from build123d import *

# Parameters (mm, degrees)
BASPROSKE_W         = 4
BASPROSKE_H         = 7.875
TOOTHCUT_DEPTH      = 12.833480046
TEETHCUTS_COUNT     = 12
TEETHCUTS_ANGLE     = 330
BORSKE_R            = 1
BORE_DEPTH          = 50.0000508
SKETCH1_R           = 3.25
SKETCH1_R_2         = 2.25
BOSS_EXTRUDE1_DEPTH = 2
SKETCH2_R           = 2
CUT_EXTRUDE1_DEPTH  = 3


with BuildPart() as part:
    # BasProSke → Base-Revolve (revolve)
    with BuildSketch(Plane(origin=(0, 0, 0), x_dir=(1, 0, 0), z_dir=(0, 1, 0)), mode=Mode.PRIVATE) as base_revolve_sk:
        with Locations((2, 3.9375)):
            Rectangle(BASPROSKE_W, BASPROSKE_H)
    revolve(base_revolve_sk.sketch.rotate(Axis((-10, 0, 0), (1, 0, 0)), 180), axis=Axis((-10, 0, 0), (1, 0, 0)))

    # TooCutSke → ToothCut (cut, through all)
    with BuildSketch(Plane(origin=(0, 0, 0), x_dir=(0, 0, -1), z_dir=(1, 0, 0))):
        with BuildLine():
            ThreePointArc((0.631439839, 5.305305014), (0, 5.34275), (-0.631439839, 5.305305014))
            ThreePointArc((-0.631439839, 5.305305014), (-0.93992237, 6.654932089), (-1.876748184, 7.674251521))
            ThreePointArc((-1.876748184, 7.674251521), (0, 7.9004), (1.876748184, 7.674251521))
            ThreePointArc((1.876748184, 7.674251521), (0.93992237, 6.654932089), (0.631439839, 5.305305014))
        make_face()
    toothcut = extrude(amount=TOOTHCUT_DEPTH, mode=Mode.SUBTRACT)

    # TeethCuts: ToothCut ×12 about axis
    teethcuts_axis = Axis((-10, 0, 0), (1, 0, 0))
    for i in range(1, TEETHCUTS_COUNT):
        add(toothcut.rotate(teethcuts_axis, i * TEETHCUTS_ANGLE / (TEETHCUTS_COUNT - 1)), mode=Mode.SUBTRACT)

    # BorSke → Bore (cut, symmetric)
    with BuildSketch(Plane(origin=(0, 0, 0), x_dir=(0, 0, -1), z_dir=(1, 0, 0))):
        with Locations(Location((0, 0, 0), (0, 0, 180))):
            Circle(BORSKE_R)
    extrude(amount=BORE_DEPTH, both=True, mode=Mode.SUBTRACT)

    # Sketch1 → Boss-Extrude1 (add)
    with BuildSketch(Plane.ZY):
        with Locations(Location((0, 0, 0), (0, 0, 180))):
            Circle(SKETCH1_R)
        Circle(SKETCH1_R_2, mode=Mode.SUBTRACT)
    extrude(amount=BOSS_EXTRUDE1_DEPTH)

    # Sketch2 → Cut-Extrude1 (cut)
    with BuildSketch(Plane(origin=(4, 0, 0), x_dir=(0, 0, -1), z_dir=(1, 0, 0))):
        Circle(SKETCH2_R)
    extrude(amount=-CUT_EXTRUDE1_DEPTH, mode=Mode.SUBTRACT)


solid = part.part
Could you check a few things on this model? Use its own coordinates, in mm. A direction names the side the tool comes from. Give positions to 0.01 mm unless a question says otherwise; leave off trailing zeros. Order: outer loops, then holes, each group sorted by start corner. A loop starts at its lowest first (then second) coordinate and runs counter-clockwise, first axis right, second up. Notation, with made-up numbers: (17, -19) -> (55, -19) arc R18 cw to (55, 10) -> close; hole circle Ø2 at (16.5, -1). An arc over 180 degrees is marked (long way). Answer in a Markdown table with one row per item. Add a question column.
Item 1: Imagine slicing it at A-A (z = 0). List the corners of the cut face in (x, y) for me.
Item 2: I'm going to push flat-ended pins straight in: P1, Ø8, axis at y = 0, z = -5, coming from the -X side; P2, Ø2, axis at y = 0.5, z = -0.5, coming from the +X side. Where does each tip first touch, or does it pass through?
Item 3: Please list where these lines run through material, in increasing order: probe 1 along Y at (x, z) = (-0.8, 0); probe 2 along Z at (x, y) = (3.2, -5); probe 3 along Y at (x, z) = (2.55, 0).
Item 4: Imagine slicing it at D-D (z = 6.75). List the corners of the cut face in (x, y) for me.
Item 5: Imagine slicing it at C-C (x = -0.8). List the corners of the cut face in (y, z) for me.
Item 6: We'd pull the mould along Y, two halves only. Please class faces 1 (the cylindrical face through (1.97, -2.51, -6.2)), 2 (the cylindrical face through (-0.986, 1.978, 2.579)): pulls with the +Y half, pulls with the -Y half, needs draft (parallel to the pull), parting line crosses it, or undercut.
Item 7: For faces 3 (the cylindrical face through (1.972, -6.235, -2.514)), 4 (the flat face through (1, -1, -1)), which set-ups out of +Z, -Z, +X, -X, +Y, -Y let a thin tool reach every point of the face, with its end or its side?
Result:
| question | item | result |
|---|---|---|
| 1 | outline | (-2, -3.25) -> (0, -3.25) -> (0, -5.34) -> (4, -5.34) -> (4, -2) -> (1, -2) -> (1, -1) -> (0, -1) -> (0, -2.25) -> (-2, -2.25) -> close; (-2, 2.25) -> (0, 2.25) -> (0, 1) -> (1, 1) -> (1, 2) -> (4, 2) -> (4, 5.34) -> (0, 5.34) -> (0, 3.25) -> (-2, 3.25) -> close |
| 2 | P1 | x = -2 |
| 2 | P2 | x = 1 |
| 3 | probe 1 | -3.25 to -2.25, 2.25 to 3.25 |
| 3 | probe 2 | -5.65 to -3.76, -2.16 to 2.16, 3.76 to 5.65 |
| 3 | probe 3 | -5.34 to -2, 2 to 5.34 |
| 4 | outline | (0, -2.48) -> (4, -2.48) -> (4, -0.99) -> (0, -0.99) -> close; (0, 0.99) -> (4, 0.99) -> (4, 2.48) -> (0, 2.48) -> close |
| 5 | outline | circle Ø6.5 at (0, 0); hole circle Ø4.5 at (0, 0) |
| 6 | face 1 | undercut |
| 6 | face 2 | parting line crosses it |
| 7 | face 3 | +X, -X |
| 7 | face 4 | +X |
